The figure shows three views and two pictorial views of one solid part (mm, origin at its lowest corner). Answer the questions. A direction names the side the tool comes from. Round coordinates to 2 decimals unless told otherwise and drop trailing zeros. Order: outer loops, then holes, each group sorted by start corner. A loop starts at its lowest first (then second) coordinate and runs counter-clockwise, first axis right, second up. Notation, with made-up numbers: M -14,-23 L -3,-23 A21 cw -3,-16 Z; hole C 37.5,28 d10. An arc over 180 degrees is marked long. Return JSON: item names as keys, results as strings.
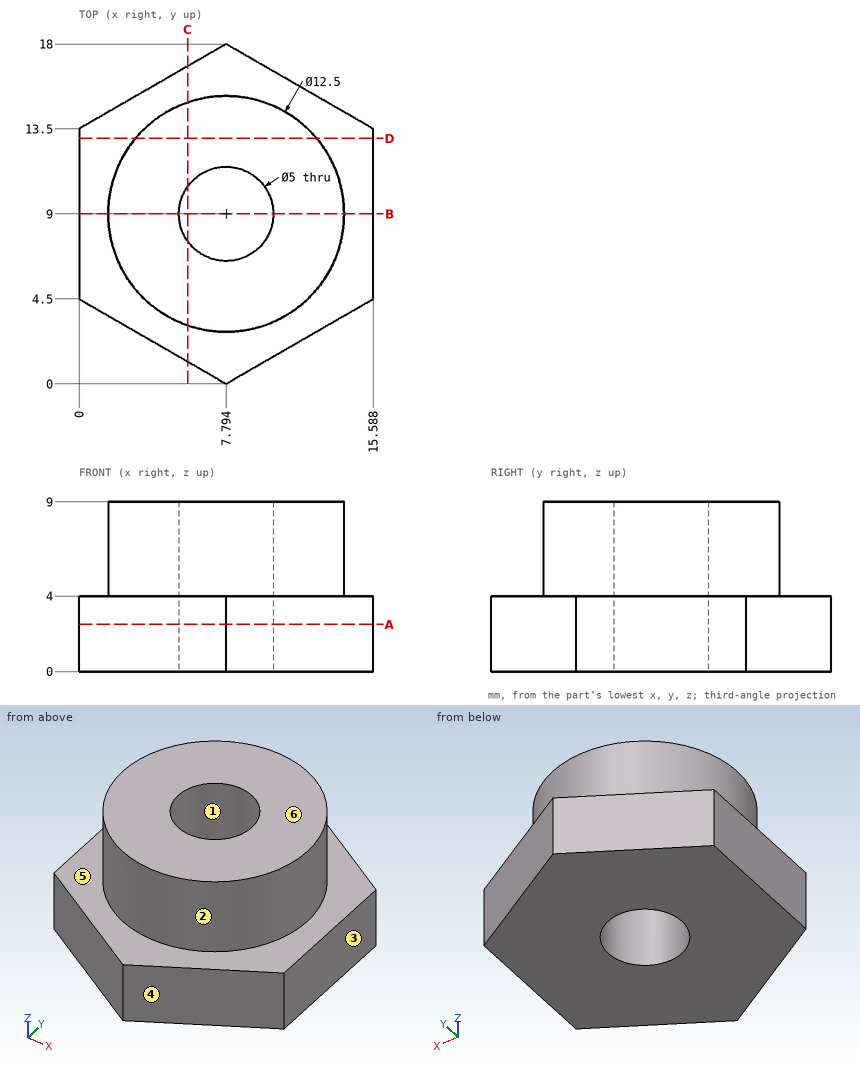
Item 1: The mould has two halves that part along Y. Classify the marked faces 1, 2, 3 and 4: pulls with the +Y half, pulls with the -Y half, needs draft (parallel to the pull), parting line crosses it, or undercut.
Output:
{"face 1": "undercut", "face 2": "parting line crosses it", "face 3": "needs draft", "face 4": "pulls with the -Y half"}
Item 2: Find section C-C (x = 5.75). Determine the outline of the cut face in (y, z).
Output:
{"outline": "M 1.18,0 L 7.56,0 L 7.56,9 L 3.09,9 L 3.09,4 L 1.18,4 Z; M 10.44,0 L 16.82,0 L 16.82,4 L 14.91,4 L 14.91,9 L 10.44,9 Z"}
Item 3: Find section D-D (y = 13). Determine the outline of the cut face in (x, z), plus the area to 3 significant figures.
Output:
{"outline": "M 0,0 L 15.59,0 L 15.59,4 L 12.6,4 L 12.6,9 L 2.99,9 L 2.99,4 L 0,4 Z", "area": "110 mm^2"}
Item 4: Find section A-A (z = 2.5). Determine the outline of the cut face in (x, y) (1 decimal), plus the area to 3 significant figures.
Output:
{"outline": "M 0,4.5 L 7.8,0 L 15.6,4.5 L 15.6,13.5 L 7.8,18 L 0,13.5 Z; hole C 7.8,9 d5", "area": "191 mm^2"}
Item 5: Consider line 1 along Z through (x, y) = (13.5, 13.5); line 2 along Y through (x, z) = (5.75, 2); line 3 along X through (y, z) = (11, 6) (1 decimal). Determine where each line is inside the solid, lowest interval first. Write a range as [from, to].
Output:
{"line 1": "z = [0, 4]", "line 2": "y = [1.18, 7.56], [10.44, 16.82]", "line 3": "x = [1.9, 6.3], [9.3, 13.7]"}
Item 6: Which of the six approach directions +Z, -Z, +X, -X, +Y, -Y give full straight-line access (tool end or side, diameter ignored) to the marked faces 5 and 6?
Output:
{"face 5": "+Z", "face 6": "+Z, +X, -X, +Y, -Y"}
Item 7: Each of these flat-tipped pins is pushed along its axis until it touches: pin 1 (1.5 mm diameter, centred on y = 13, z = 5, fed in from +X); pin 2 (3 mm diameter, centred on x = 5.5, z = 5, fed in from -Y); pin 3 (3 mm diameter, centred on y = 16, z = 1.5, fed in from -X). Where does it stop, or does it pass through?
Output:
{"pin 1": "stops at x = 13.13", "pin 2": "stops at y = 0.68", "pin 3": "stops at x = 1.73"}
Item 8: Find section B-B (y = 9). Determine the outline of the cut face in (x, z) (1 decimal).
Output:
{"outline": "M 0,0 L 5.3,0 L 5.3,9 L 1.5,9 L 1.5,4 L 0,4 Z; M 10.3,0 L 15.6,0 L 15.6,4 L 14,4 L 14,9 L 10.3,9 Z"}
